Source: three-view drawing plus pictorial views. Frame: mm from the lowest corner of the part. A direction names the side the tool comes from. Give positions to 0.01 mm unless a question says otherwise; leave off trailing zeros. Loops run counter-clockwise (first coordinate to the right, second up) from the corner with the lowest first, then second, coordinate; pieces in that order, holes last. Notation, with made-up numbers: (63, 52) -> (95, 52) arc R13 cw to (95, 60) -> close; hole circle Ø4 at (48.5, 6.5). An arc over 180 degrees is marked (long way). Answer in a Markdown table with one row per item. Add a question column.
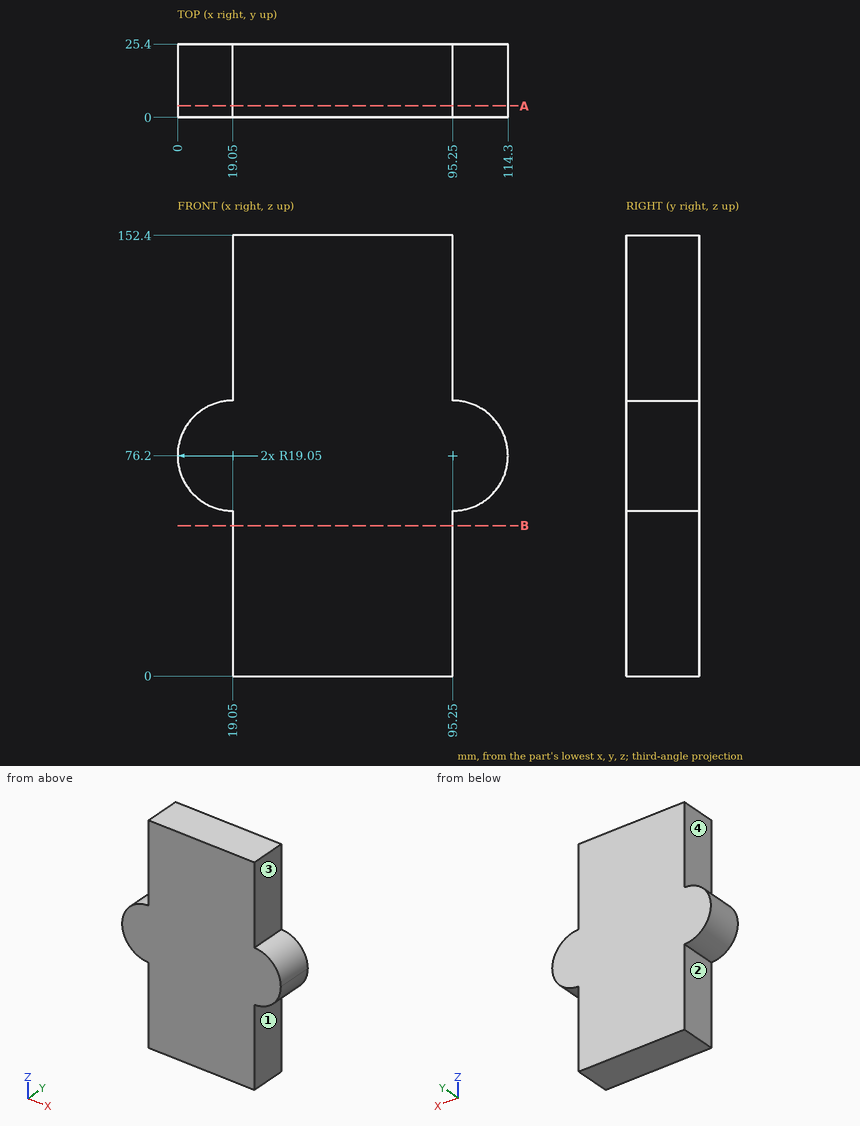
(1) Pin query (flat end, axial travel): pin 1 Ø12.5 at (y, z) = (10, 122) entering from -X; pin 2 Ø5 at (y, z) = (16, 20.5) entering from +X; pin 3 Ø1.5 at (y, z) = (17, 72.5) entering from +X. Return the tip coordinate at first contact, or that it passes through.
(2) Reachability of the marked faces 1, 2, 3 and 4 from +Z, -Z, +X, -X, +Y, -Y: full face, straight path, thin tool, end or side. Return the list, or none.
(3) Material intervals for line 1 along X through (y, z) = (2.25, 29); line 2 along Z through (x, y) = (9.5, 17.75); line 3 along X through (y, z) = (6.5, 79.5), sorted ascending. Write a range as from..to.
(4) Cut plane A-A on y = 4. Return the cut outline in (x, z), then the cut area to 3 significant figures.
(5) Cut plane B-B on z = 52. Return the cut outline in (x, y).
Answer list:
| question | item | result |
|---|---|---|
| 1 | pin 1 | stops at x = 19.05 |
| 1 | pin 2 | stops at x = 95.25 |
| 1 | pin 3 | stops at x = 114.07 |
| 2 | face 1 | -Z, +X, +Y, -Y |
| 2 | face 2 | -Z, -X, +Y, -Y |
| 2 | face 3 | +Z, +X, +Y, -Y |
| 2 | face 4 | +Z, -X, +Y, -Y |
| 3 | line 1 | x = 19.05..95.25 |
| 3 | line 2 | z = 59.72..92.68 |
| 3 | line 3 | x = 0.29..114.01 |
| 4 | outline | (19.05, 0) -> (95.25, 0) -> (95.25, 57.15) arc R19.05 ccw to (95.25, 95.25) -> (95.25, 152.4) -> (19.05, 152.4) -> (19.05, 95.25) arc R19.05 ccw to (19.05, 57.15) -> close |
| 4 | area | 12,800 mm² |
| 5 | outline | (19.05, 0) -> (95.25, 0) -> (95.25, 25.4) -> (19.05, 25.4) -> close |
